Work out the finished part from the listing and answer in its coordinate system (mm). A direction names the side the tool comes from. Coordinates: 2 decimals unless noted, no trailing zeros. Order: outer loops, then holes, each group sorted by start corner. A loop starts at its lowest first (then second) coordinate and runs counter-clockwise, first axis right, second up.
```python
from build123d import *

# Parameters (mm, degrees)
BOSS_EXTRUDE1_DEPTH = 10
SKETCH2_R           = 4.1
CUT_EXTRUDE1_DEPTH  = 29.284271247
CUT_EXTRUDE2_DEPTH  = 8
BOSS_EXTRUDE2_START = 10
SKETCH4_R           = 7.5
SKETCH4_R_2         = 4.1
BOSS_EXTRUDE2_DEPTH = 10
FILLET1_R           = 10


with BuildPart() as part:
    # Sketch1 → Boss-Extrude1 (new body)
    with BuildSketch(Plane(origin=(0, 0, 0), x_dir=(1, 0, 0), z_dir=(0, 1, 0))):
        Polygon((-10, 17.320508076), (-20, 0), (-10, -17.320508076), (10, -17.320508076), (20, 0), (10, 17.320508076), align=None)
    extrude(amount=BOSS_EXTRUDE1_DEPTH)

    # Sketch2 → Cut-Extrude1 (cut, through all)
    with BuildSketch(Plane(origin=(0, 10, 0), x_dir=(1, 0, 0), z_dir=(0, 1, 0))):
        with Locations(Location((0, 0, 0), (0, 0, 270))):
            Circle(SKETCH2_R)
    extrude(amount=-CUT_EXTRUDE1_DEPTH, mode=Mode.SUBTRACT)

    # Sketch3 → Cut-Extrude2 (cut)
    with BuildSketch(Plane.XZ):
        Polygon((7.5, 0), (3.75, 6.495190528), (-3.75, 6.495190528), (-7.5, 0), (-3.75, -6.495190528), (3.75, -6.495190528), align=None)
    extrude(amount=-CUT_EXTRUDE2_DEPTH, mode=Mode.SUBTRACT)

    # Sketch4 → Boss-Extrude2 (add)
    with BuildSketch(Plane(origin=(0, 10, 0), x_dir=(1, 0, 0), z_dir=(0, 1, 0)).offset(BOSS_EXTRUDE2_START)):
        with Locations(Location((0, 0, 0), (0, 0, 270))):
            Circle(SKETCH4_R)
        with Locations(Location((0, 0, 0), (0, 0, 270))):
            Circle(SKETCH4_R_2, mode=Mode.SUBTRACT)
    extrude(amount=-BOSS_EXTRUDE2_DEPTH)

    # Fillet1
    fillet1_edges = [part.edges().sort_by_distance(p)[0] for p in [
        (0, 10, -7.5),
    ]]
    fillet(fillet1_edges, radius=FILLET1_R - 0.0001)  # a hair under: the kernel refuses the full size


solid = part.part
```
1. Flat-ended cylindrical pins translate along their axes: pin 1 (9.5 mm diameter, centred on x = 0, z = 0, fed in from -Y); pin 2 (3 mm diameter, centred on x = 6, z = 15.5, fed in from +Y); pin 3 (3 mm diameter, centred on x = 9.5, z = -15, fed in from +Y). Find the tip coordinate at first contact, or state that the pin passes through.
2. The part is cut by section A-A (y = 5.5). Determine the outline of the cut face in (x, z), plus the area to 3 significant figures.
3. Consider probe 1 along Z at (x, y) = (-1, 15); probe 2 along Y at (x, z) = (16, -6.5); probe 3 along X at (y, z) = (6, -2.5). Determine where each line is inside the solid, lowest interval first.
4. The mould has two halves that part along Z. Classify faces 6 (the flat face through (-18, 10, 0)), 7 (the flat face through (-14.93, 4.93, -8.78)), 8 (the flat face through (5.6, 3.94, -3.29)): released by +Z, released by -Z, zero draft, split by the parting line, or undercut.
5. For faces 1 (the flat face through (9, 10, -16)), 2 (the flat face through (3.2, 8, 3)), 3 (the flat face through (0, 5, -17.321)), 4 (the flat face through (9, 10, 16)), 5 (the flat face through (-9, 10, 16)), determine the directions among +Z, -Z, +X, -X, +Y, -Y from which every point of the face is accessible in a straight line to the end or side of a thin tool.
Worked out:
1. pin 1: stops at y = 8
1. pin 2: stops at y = 10.29
1. pin 3: stops at y = 10.08
2. outline: (-20, 0) - (-10, -17.32) - (10, -17.32) - (20, 0) - (10, 17.32) - (-10, 17.32) - close; hole (-7.5, 0) - (-3.75, -6.5) - (3.75, -6.5) - (7.5, 0) - (3.75, 6.5) - (-3.75, 6.5) - close
2. area: 893 mm2
3. probe 1: z = -8.78 to -3.98, 3.98 to 8.78
3. probe 2: y = 0 to 10
3. probe 3: x = -18.56 to -6.06, 6.06 to 18.56
4. face 6: zero draft
4. face 7: released by -Z
4. face 8: undercut
5. face 1: -Z, +X, +Y
5. face 2: -Y
5. face 3: -Z, +X, -X, +Y, -Y
5. face 4: +Z, +X, +Y
5. face 5: +Z, -X, +Y
